The listing builds one solid part. Answer for the finished solid, in the listing's coordinates (mm). A direction names the side the tool comes from. Round coordinates to 2 decimals unless told otherwise and drop trailing zeros. Loops run counter-clockwise (first coordinate to the right, second up) from the corner with the lowest first, then second, coordinate; pieces in that order, holes last. Notation, with made-up numbers: (-15, -22) -> (6, -22) arc R24 cw to (6, -1) -> close; hole circle Ø8 at (-37.5, 32). An arc over 180 degrees is marked (long way). Use a Markdown table: item, result. Add a question column.
Q1. Section C-C on x = 6.5 is taken. Give the vertices of the cut face in (y, z).
Q2. Consider line 1 (Y direction, x = 83, z = 0); line 2 (Z direction, x = 6.5, y = 5.25); line 3 (X direction, y = 0.75, z = 4.5). Determine where each line is inside the solid, lowest interval first.
Q3. Section B-B on y = 3.5 is taken. Give the vertices of the cut face in (x, z), then the cut area to 3 significant figures.
Q4. Given pin 1 Ø2.5 at (x, y) = (2.29, 3.5) entering from -Z; pin 2 Ø4 at (y, z) = (3, 29.5) entering from -X; pin 3 Ø2 at (x, y) = (-1.5, 4) entering from -Z; pin 4 Ø4 at (y, z) = (3, 25) entering from +X, each flat-ended and moving along its own axis, determine where each tip first touches the part or whether it passes through.
Q5. Section D-D on z = 51.5 is taken. Give the vertices of the cut face in (x, y).
Q6. Section A-A on z = 0.75 is taken. Give the vertices of the cut face in (x, y).
Q7. Which of the six approach directions +Z, -Z, +X, -X, +Y, -Y give full straight-line access (tool end or side, diameter ignored) to faces 1 (the flat face through (66.9, 3.5, 27.8)), 2 (the flat face through (0, 3, 81.15))?
Q8. For a pull along Y with two mould halves and no side action, classify faces 3 (the flat face through (47, 0, 44)), 4 (the flat face through (2.4, 1.9, 87.15)), 5 (the cylindrical face through (82.481, 2.214, 1.419)) as released by +Y, released by -Y, zero draft, split by the parting line, or undercut.
from build123d import *

# Parameters (mm, degrees)
BOSS_EXTRUDE1_DEPTH = 7
SKETCH14_R          = 1.45
CUT_EXTRUDE1_DEPTH  = 10
SKETCH15_R          = 1.45
CUT_EXTRUDE2_DEPTH  = 10


with BuildPart() as part:
    # Sketch12 → Boss-Extrude1 (new body)
    with BuildSketch(Plane(origin=(0, 0, 0), x_dir=(1, 0, 0), z_dir=(0, 1, 0))):
        Polygon((85.522563955, 6.5), (85.522563955, -8.5), (47.695057641, -47.704563591), (9.792563955, -87.15), (-5.207436045, -87.15), (-5.207436045, -81.15), (7.792563955, -81.15), (43.657563955, -43.825), (79.522563955, -6.5), (79.522563955, 6.5), align=None)
    extrude(amount=BOSS_EXTRUDE1_DEPTH)

    # Sketch14 → Cut-Extrude1 (cut)
    with BuildSketch(Plane(origin=(0, 0, 81.15), x_dir=(-1, 0, 0), z_dir=(0, 0, -1))):
        with Locations((-2.292563955, 3.5)):
            Circle(SKETCH14_R)
    extrude(amount=-CUT_EXTRUDE1_DEPTH, mode=Mode.SUBTRACT)

    # Sketch15 → Cut-Extrude2 (cut)
    with BuildSketch(Plane.ZY.offset(-79.522563955)):
        with Locations((0.75, 3.5)):
            Circle(SKETCH15_R)
    extrude(amount=-CUT_EXTRUDE2_DEPTH, mode=Mode.SUBTRACT)


solid = part.part
Checked values:
| question | item | result |
|---|---|---|
| 1 | outline | (0, 81.15) -> (7, 81.15) -> (7, 87.15) -> (0, 87.15) -> close |
| 2 | line 1 | y = 0 to 2.26, 4.74 to 7 |
| 2 | line 2 | z = 81.15 to 87.15 |
| 2 | line 3 | x = 79.52 to 85.52 |
| 3 | outline | (-5.21, 81.15) -> (0.84, 81.15) -> (0.84, 87.15) -> (-5.21, 87.15) -> close; (3.74, 81.15) -> (7.79, 81.15) -> (79.52, 6.5) -> (79.52, 2.2) -> (85.52, 2.2) -> (85.52, 8.5) -> (47.7, 47.7) -> (9.79, 87.15) -> (3.74, 87.15) -> close; (79.52, -6.5) -> (85.52, -6.5) -> (85.52, -0.7) -> (79.52, -0.7) -> close |
| 3 | area | 732 mm2 |
| 4 | pin 1 | passes through |
| 4 | pin 2 | stops at x = 55.5 |
| 4 | pin 3 | stops at z = 81.15 |
| 4 | pin 4 | stops at x = 71.53 |
| 5 | outline | (36.28, 0) -> (44.05, 0) -> (44.05, 7) -> (36.28, 7) -> close |
| 6 | outline | (79.52, 0) -> (85.52, 0) -> (85.52, 2.05) -> (79.52, 2.05) -> close; (79.52, 4.95) -> (85.52, 4.95) -> (85.52, 7) -> (79.52, 7) -> close |
| 7 | face 1 | +Z, +X, +Y, -Y |
| 7 | face 2 | -Z, -X, +Y, -Y |
| 8 | face 3 | released by -Y |
| 8 | face 4 | zero draft |
| 8 | face 5 | undercut |
